Source: CAD feature listing. Evaluate the final solid. Frame: model axes, mm. Round coordinates to 2 decimals unless told otherwise and drop trailing zeros.
(1) Material intervals for probe 1 along X at (y, z) = (45.5, 0.3); probe 2 along Y at (x, z) = (119.5, 2.7); probe 3 along Y at (x, z) = (203, 1.7), sorted ascending.
(2) Mould query, pull axis X, two halves, no side actions, for faces 1 (the flat face through (140.957, 36.225, 1.565)), 2 (the flat face through (100, 46, 0)), 3 (the flat face through (55.48, 54.66, 1.57)). Classes: pulls with the +X half, pulls with the -X half, needs draft (parallel to the pull), parting line crosses it, or undercut.
(3) First-contact query: pin 1 Ø1.6 at (y, z) = (9, 2) entering from -X; pin 2 Ø1.2 at (y, z) = (4.5, 1) entering from +X; pin 3 Ø1.2 at (x, z) = (39.5, 1) entering from -Y. Flat tips, straight axial feed; report the tip coordinate or a pass-through.
```python
from build123d import *

# Parameters (mm, degrees)
BOSS_EXTRUDE1_DEPTH = 3.175
SKETCH3_W           = 8
SKETCH3_H           = 3.175
BOSS_EXTRUDE2_DEPTH = 3.175
CUT_EXTRUDE1_DEPTH  = 295.302026077


with BuildPart() as part:
    # Sketch2 → Boss-Extrude1 (new body)
    with BuildSketch(Plane.XY):
        with BuildLine():
            Line((0, 0), (71.821224644, 0))
            add(Edge.make_bspline(
                [(113.265068403, 31.345085694), (88.49122235, 22.260941948), (71.821224644, 0)],
                knots=[0, 0, 0, 1, 1, 1], degree=2))
            Line((113.265068403, 31.345085694), (169.435947463, 41.242848876))
            add(Edge.make_bspline(
                [(134.041587412, 44.130878692), (151.78543129, 43.239991284), (169.435947463, 41.242848876)],
                knots=[0, 0, 0, 1, 1, 1], degree=2))
            add(Edge.make_bspline(
                [(149.664509426, 59.598208841), (133.564564098, 59.446315657), (134.041587412, 44.130878692)],
                knots=[0, 0, 0, 1, 1, 1], degree=2))
            Line((149.664509426, 59.598208841), (149.685676558, 60.6678268))
            Line((149.685676558, 60.6678268), (160.696312712, 64.401472217))
            add(Edge.make_bspline(
                [(160.696312712, 64.401472217), (156.792494019, 64.794773064), (153.080099679, 63.60900386)],
                knots=[0, 0, 0, 1, 1, 1], degree=2))
            add(Edge.make_bspline(
                [(153.080099679, 63.60900386), (153.21581852, 65.543109048), (155.855294119, 65.154686594)],
                knots=[0, 0, 0, 1, 1, 1], degree=2))
            add(Edge.make_bspline(
                [(155.855294119, 65.154686594), (168.070276532, 67.039683705), (180.482777211, 66.945466473)],
                knots=[0, 0, 0, 1, 1, 1], degree=2))
            add(Edge.make_bspline(
                [(180.482777211, 66.945466473), (171.187708605, 72.067803505), (182.417352528, 74.400222782)],
                knots=[0, 0, 0, 1, 1, 1], degree=2))
            add(Edge.make_bspline(
                [(182.417352528, 74.400222782), (202.456511943, 79.784692432), (223.217555695, 81.328050857)],
                knots=[0, 0, 0, 1, 1, 1], degree=2))
            add(Edge.make_bspline(
                [(275.233904512, 101.469551945), (286.543816843, 98.715878969), (194.296992898, 91.024580871), (223.217555695, 81.328050857)],
                knots=[0, 0, 0, 0, 1, 1, 1, 1], degree=3))
            add(Edge.make_bspline(
                [(275.233904512, 101.469551945), (174.061816158, 103.537553967), (81.190900328, 63.774105239)],
                knots=[0, 0, 0, 1, 1, 1], degree=2))
            add(Edge.make_bspline(
                [(81.190900328, 63.774105239), (88.381783724, 65.999307209), (95.832537282, 65.154686594)],
                knots=[0, 0, 0, 1, 1, 1], degree=2))
            add(Edge.make_bspline(
                [(95.832537282, 65.154686594), (96.183075401, 62.049994654), (93.003333324, 60.309886397)],
                knots=[0, 0, 0, 1, 1, 1], degree=2))
            add(Edge.make_bspline(
                [(93.003333324, 60.309886397), (79.982990497, 52.245061614), (64.511543782, 52.550984526)],
                knots=[0, 0, 0, 1, 1, 1], degree=2))
            add(Edge.make_bspline(
                [(64.511543782, 52.550984526), (59.095264392, 53.626200699), (67.149577001, 58.996482621)],
                knots=[0, 0, 0, 1, 1, 1], degree=2))
            Line((67.149577001, 58.996482621), (43.476372801, 50.196200023))
            add(Edge.make_bspline(
                [(43.476372801, 50.196200023), (39.603225427, 49.243326926), (42.576727954, 52.611474892)],
                knots=[0, 0, 0, 1, 1, 1], degree=2))
            add(Edge.make_bspline(
                [(42.576727954, 52.611474892), (5.440445948, 36.121326287), (0, 0)],
                knots=[0, 0, 0, 1, 1, 1], degree=2))
        make_face()
    extrude(amount=BOSS_EXTRUDE1_DEPTH)

    # Sketch3 → Boss-Extrude2 (add)
    with BuildSketch(Plane.XY.offset(3.175)):
        with Locations((21, -1.5875)):
            Rectangle(SKETCH3_W, SKETCH3_H)
        with Locations((51, -1.5875)):
            Rectangle(SKETCH3_W, SKETCH3_H)
    extrude(amount=-BOSS_EXTRUDE2_DEPTH)

    # Sketch4 → Cut-Extrude1 (cut, through all)
    with BuildSketch(Plane.XY.offset(3.175)):
        Polygon((28.5, 4), (28.5, 0), (31.5, 0), (31.5, 4), (33.05, 4), (33.05, 6.4), (31.5, 6.4), (31.5, 12.825), (28.5, 12.825), (28.5, 6.4), (26.95, 6.4), (26.95, 4), align=None)
        Polygon((40.5, 4), (40.5, 0), (43.5, 0), (43.5, 4), (45.05, 4), (45.05, 6.4), (43.5, 6.4), (43.5, 12.825), (40.5, 12.825), (40.5, 6.4), (38.95, 6.4), (38.95, 4), align=None)
    extrude(amount=-CUT_EXTRUDE1_DEPTH, mode=Mode.SUBTRACT)


solid = part.part
```
Output values:
1. probe 1: x = 29.4 to 134.03
1. probe 2: y = 32.44 to 78.28
1. probe 3: y = 78.89 to 97.48
2. face 1: pulls with the +X half
2. face 2: needs draft
2. face 3: undercut
3. pin 1: stops at x = 1.71
3. pin 2: stops at x = 75.89
3. pin 3: stops at y = 0
